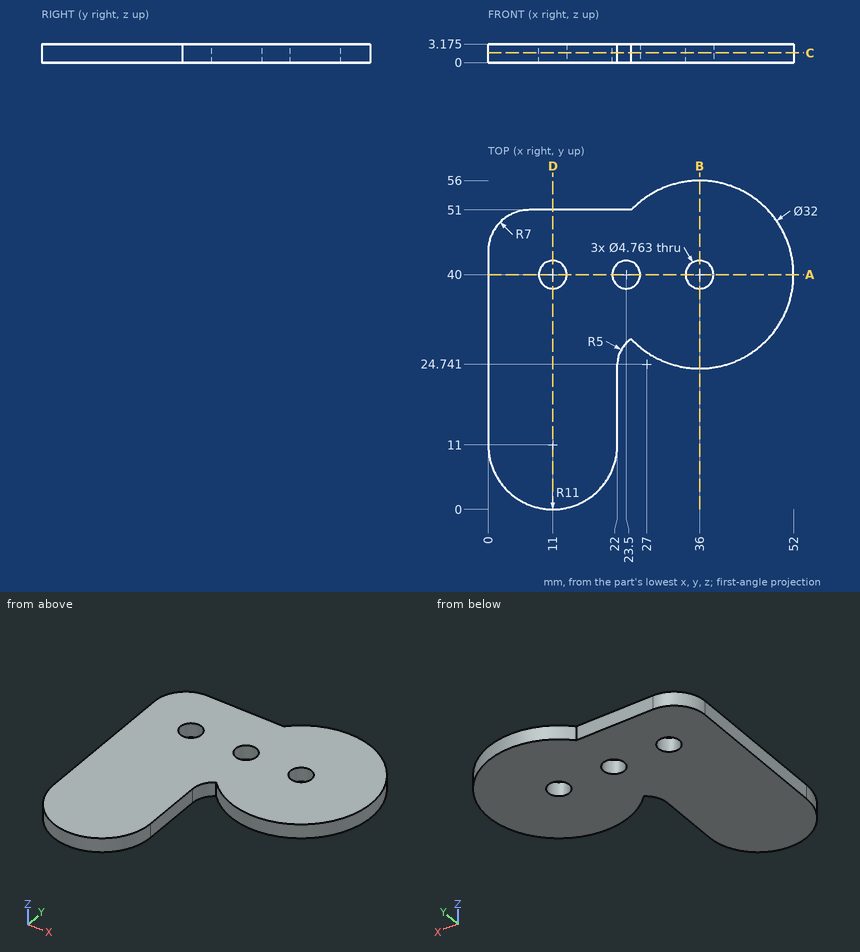
Could you check a few things on this drawing? It's one solid part, dimensions in mm from its lowest x, y, z. Coordinates: 2 decimals unless noted, no trailing zeros. Order: outer loops, then holes, each group sorted by start corner. A loop starts at its lowest first (then second) coordinate and runs counter-clockwise, first axis right, second up. Notation, with made-up numbers: (-34.5, 1) -> (-25.5, 1) arc R6 ccw to (-25.5, 12) -> close; hole circle Ø4 at (27.5, 67). An arc over 180 degrees is marked (long way). Answer in a Markdown table with one row per item.
(1) I want a section at C-C on z = 1.65. List the corners of the cut face in (x, y) for me.
Answer key:
| item | result |
|---|---|
| outline | (0, 11) arc R11 ccw to (22, 11) -> (22, 24.74) arc R5 cw to (24.38, 29) arc R16 ccw (long way) to (24.38, 51) -> (7, 51) arc R7 ccw to (0, 44) -> close; hole circle Ø4.76 at (11, 40); hole circle Ø4.76 at (23.5, 40); hole circle Ø4.76 at (36, 40) |
(2) Please list where these lines run through material, in increasing order: probe 1 along Y at (x, z) = (36, 2.35); probe 2 along X at (y, z) = (41, 1.05); probe 3 along Y at (x, z) = (23.5, 1.95).
Answer key:
| item | result |
|---|---|
| probe 1 | 24 to 37.62, 42.38 to 56 |
| probe 2 | 0 to 8.84, 13.16 to 21.34, 25.66 to 33.84, 38.16 to 51.97 |
| probe 3 | 28.31 to 37.62, 42.38 to 51 |
(3) I want a section at B-B on x = 36. List the corners of the cut face in (y, z) for me (1 decimal).
Answer key:
| item | result |
|---|---|
| outline | (24, 0) -> (37.6, 0) -> (37.6, 3.2) -> (24, 3.2) -> close; (42.4, 0) -> (56, 0) -> (56, 3.2) -> (42.4, 3.2) -> close |
(4) I want a section at A-A on y = 40. List the corners of the cut face in (x, z) for me (1 decimal), then the cut area to 3 significant figures.
Answer key:
| item | result |
|---|---|
| outline | (0, 0) -> (8.6, 0) -> (8.6, 3.2) -> (0, 3.2) -> close; (13.4, 0) -> (21.1, 0) -> (21.1, 3.2) -> (13.4, 3.2) -> close; (25.9, 0) -> (33.6, 0) -> (33.6, 3.2) -> (25.9, 3.2) -> close; (38.4, 0) -> (52, 0) -> (52, 3.2) -> (38.4, 3.2) -> close |
| area | 120 mm^2 |
(5) I want a section at D-D on x = 11. List the corners of the cut face in (y, z) for me (1 decimal).
Answer key:
| item | result |
|---|---|
| outline | (0, 0) -> (37.6, 0) -> (37.6, 3.2) -> (0, 3.2) -> close; (42.4, 0) -> (51, 0) -> (51, 3.2) -> (42.4, 3.2) -> close |
